Geometry check sheet. Reference: the model listing, model coordinates, mm. Face numbers are marked on the shaded views. Give positions to 0.01 mm unless a question says otherwise; leave off trailing zeros. Order: outer loops, then holes, each group sorted by start corner. A loop starts at its lowest first (then second) coordinate and runs counter-clockwise, first axis right, second up. Notation, with made-up numbers: M -28,54 L -18,54 A35 cw -18,86 Z; hole C 6,70 d10. An arc over 180 degrees is marked long. Answer as CSV lines item,"result".
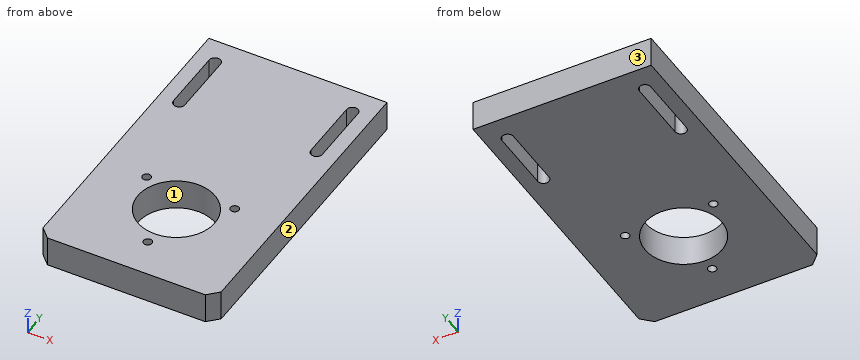
from build123d import *

# Parameters (mm, degrees)
EXTRUDE_1_DEPTH     = 12
SKETCH_2_R          = 15.1
CUT_EXTRUDE_1_DEPTH = 90.199215243
M4X0_7_1_D          = 3.3
CUT_EXTRUDE_2_DEPTH = 90.199215243


with BuildPart() as part:
    # 草图1 → 凸台-拉伸1 (new body)
    with BuildSketch(Plane.XY):
        Polygon((-38.5, -42.5), (23.5, -42.5), (27.5, -38.5), (27.5, 77.5), (-42.5, 77.5), (-42.5, -38.5), align=None)
    extrude(amount=EXTRUDE_1_DEPTH)

    # 草图2 → 切除-拉伸1 (cut, through all)
    with BuildSketch(Plane.XY.offset(12)):
        with Locations((-7.5, -7.5)):
            Circle(SKETCH_2_R)
    extrude(amount=-CUT_EXTRUDE_1_DEPTH, mode=Mode.SUBTRACT)

    # M4x0.7 螺纹孔1 (through all)
    with Locations(Plane.XY.offset(12)):
        with Locations((-7.5, -27.5), (-24.820508076, 2.5), (9.820508076, 2.5)):
            Hole(M4X0_7_1_D / 2)

    # 草图7 → 切除-拉伸2 (cut, through all)
    with BuildSketch(Plane.XY.offset(12)):
        with BuildLine():
            Line((-32.25, 67.5), (-32.25, 42.5))
            ThreePointArc((-32.25, 42.5), (-34.5, 40.25), (-36.75, 42.5))
            Line((-36.75, 42.5), (-36.75, 67.5))
            ThreePointArc((-36.75, 67.5), (-34.5, 69.75), (-32.25, 67.5))
        make_face()
        with BuildLine():
            Line((17.25, 67.5), (17.25, 42.5))
            ThreePointArc((17.25, 42.5), (19.5, 40.25), (21.75, 42.5))
            Line((21.75, 42.5), (21.75, 67.5))
            ThreePointArc((21.75, 67.5), (19.5, 69.75), (17.25, 67.5))
        make_face()
    extrude(amount=-CUT_EXTRUDE_2_DEPTH, mode=Mode.SUBTRACT)


solid = part.part
(1) Section check A-A on y = -7.5. Enter the section's corners in (x, z).
The answers:
outline,"M -42.5,0 L -22.6,0 L -22.6,12 L -42.5,12 Z; M 7.6,0 L 27.5,0 L 27.5,12 L 7.6,12 Z"
(2) Draft check along X on the marked faces 1, 2 and 3. Enter one of: +X half, -X half, draft (parallel to the pull), parting line (faces both ways), or undercut.
The answers:
face 1,"undercut"
face 2,"+X half"
face 3,"draft"
(3) Section check B-B on x = 19.5. Enter the section's corners in (y, z).
The answers:
outline,"M -42.5,0 L 40.25,0 L 40.25,12 L -42.5,12 Z; M 69.75,0 L 77.5,0 L 77.5,12 L 69.75,12 Z"
(4) Section check D-D on x = -7.5. Enter the section's corners in (y, z), then the cut area to 3 significant figures.
The answers:
outline,"M -42.5,0 L -29.15,0 L -29.15,12 L -42.5,12 Z; M -25.85,0 L -22.6,0 L -22.6,12 L -25.85,12 Z; M 7.6,0 L 77.5,0 L 77.5,12 L 7.6,12 Z"
area,"1,040 mm2"
(5) Gauge pin test, flat end, axial feed: P1, Ø5.5, axis at x = -7.5, y = -27.5, coming from the -Z side. Record the tip position at first contact, or that the pin passes through.
The answers:
P1,"stops at z = 0"
(6) Material ranges on line 1 (X direction, y = 52, z = 6.75); line 2 (Y direction, x = -7.5, z = 7.5); line 3 (Y direction, x = 10, z = 0.5), recorded low to high.
The answers:
line 1,"x = -42.5 to -36.75, -32.25 to 17.25, 21.75 to 27.5"
line 2,"y = -42.5 to -29.15, -25.85 to -22.6, 7.6 to 77.5"
line 3,"y = -42.5 to 0.86, 4.14 to 77.5"
(7) Section check C-C on z = 8. Enter the section's corners in (x, y).
The answers:
outline,"M -42.5,-38.5 L -38.5,-42.5 L 23.5,-42.5 L 27.5,-38.5 L 27.5,77.5 L -42.5,77.5 Z; hole M -36.75,42.5 A2.25 ccw -32.25,42.5 L -32.25,67.5 A2.25 ccw -36.75,67.5 Z; hole C -24.82,2.5 d3.3; hole C -7.5,-7.5 d30.2; hole C -7.5,-27.5 d3.3; hole C 9.82,2.5 d3.3; hole M 17.25,42.5 A2.25 ccw 21.75,42.5 L 21.75,67.5 A2.25 ccw 17.25,67.5 Z"
